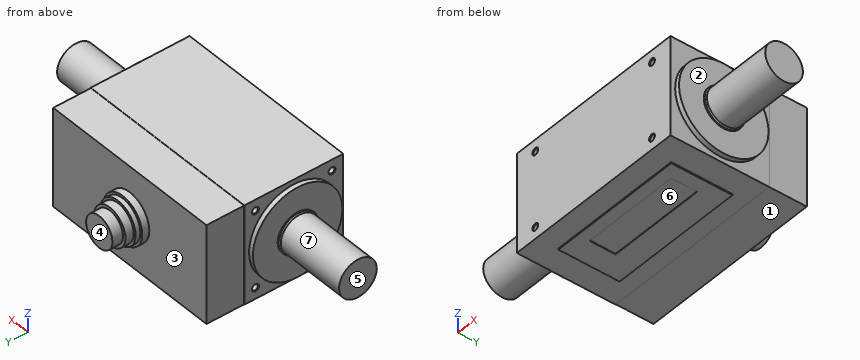
```python
from build123d import *

# Parameters (mm, degrees)
SKETCH1_W                = 79
SKETCH1_H                = 42
BOSS_EXTRUDE1_DEPTH      = 42
SKETCH2_W                = 78.8
SKETCH2_H                = 41.8
BOSS_EXTRUDE2_DEPTH      = 16
SKETCH3_W                = 58
SKETCH3_H                = 26
BOSS_EXTRUDE3_DEPTH      = 0.5
SKETCH4_W                = 42
SKETCH4_H                = 11
CUT_EXTRUDE1_DEPTH       = 0.25
M2_CLEARANCE_HOLE1_D     = 2.459
M2_CLEARANCE_HOLE1_DEPTH = 6.9
M2_CLEARANCE_HOLE1_TIP   = 0.709852156
M2_CLEARANCE_HOLE2_D     = 2.459
M2_CLEARANCE_HOLE2_DEPTH = 7.2
M2_CLEARANCE_HOLE2_TIP   = 0.709852156
CHAMFER1_SIZE            = 0.2705


with BuildPart() as part:
    # Sketch1 → Boss-Extrude1 (new body)
    with BuildSketch(Plane(origin=(0, 21, 0), x_dir=(1, 0, 0), z_dir=(0, 1, 0))):
        Rectangle(SKETCH1_W, SKETCH1_H)
    extrude(amount=-BOSS_EXTRUDE1_DEPTH)

    # Sketch2 → Boss-Extrude2 (add)
    with BuildSketch(Plane(origin=(0, 21, 0), x_dir=(-1, 0, 0), z_dir=(0, 1, 0))):
        Rectangle(SKETCH2_W, SKETCH2_H)
    extrude(amount=BOSS_EXTRUDE2_DEPTH)

    # Sketch3 → Boss-Extrude3 (add)
    with BuildSketch(Plane(origin=(0, 0, -21), x_dir=(-1, 0, 0), z_dir=(0, 0, -1))):
        with Locations((0, 1)):
            Rectangle(SKETCH3_W, SKETCH3_H)
    extrude(amount=BOSS_EXTRUDE3_DEPTH)

    # Sketch4 → Cut-Extrude1 (cut)
    with BuildSketch(Plane(origin=(0, 0, -21.5), x_dir=(-1, 0, 0), z_dir=(0, 0, -1))):
        with Locations((-2, -1.5)):
            Rectangle(SKETCH4_W, SKETCH4_H)
    extrude(amount=-CUT_EXTRUDE1_DEPTH, mode=Mode.SUBTRACT)

    # Sketch5 → Revolve1 (revolve)
    with BuildSketch(Plane(origin=(0, 0, 0), x_dir=(-1, 0, 0), z_dir=(0, 0, -1)), mode=Mode.PRIVATE) as revolve1_sk:
        Polygon((-10, 37), (0, 37), (0, 50), (-6.75, 50), (-6.75, 45.5), (-8, 45.5), (-8, 42), (-9, 42), (-9, 40), (-10, 40), align=None)
    revolve(revolve1_sk.sketch.rotate(Axis((0, 37, 0), (0, 1, 0)), 270), axis=Axis((0, 37, 0), (0, 1, 0)))

    # Sketch6 → Revolve2 (revolve)
    with BuildSketch(Plane.XY, mode=Mode.PRIVATE) as revolve2_sk:
        Polygon((39.5, 19), (39.5, 0), (72.5, 0), (72.5, 8), (42.5, 8), (42, 8.5), (41.5, 8.5), (41.5, 19), align=None)
    revolve(revolve2_sk.sketch.rotate(Axis((39.5, 0, 0), (1, 0, 0)), 270), axis=Axis((39.5, 0, 0), (1, 0, 0)))

    # Sketch7 → Revolve3 (revolve)
    with BuildSketch(Plane.XY, mode=Mode.PRIVATE) as revolve3_sk:
        Polygon((-72.5, 8), (-72.5, 0), (-39.5, 0), (-39.5, 19), (-41.5, 19), (-41.5, 8.5), (-42, 8.5), (-42.5, 8), align=None)
    revolve(revolve3_sk.sketch.rotate(Axis((-72.5, 0, 0), (1, 0, 0)), 270), axis=Axis((-72.5, 0, 0), (1, 0, 0)))

    # M2 Clearance Hole1
    with Locations(Plane.ZY.offset(39.5)):
        with Locations((-16.263455967, 16.263455967), (16.263455967, 16.263455967), (16.263455967, -16.263455967), (-16.263455967, -16.263455967)):
            Hole(M2_CLEARANCE_HOLE1_D / 2, depth=M2_CLEARANCE_HOLE1_DEPTH)
            with Locations((0, 0, -(M2_CLEARANCE_HOLE1_DEPTH + M2_CLEARANCE_HOLE1_TIP / 2))):  # 120° drill point
                Cone(0, M2_CLEARANCE_HOLE1_D / 2, M2_CLEARANCE_HOLE1_TIP, mode=Mode.SUBTRACT)

    # M2 Clearance Hole2
    with Locations(Plane.XZ.offset(21)):
        with Locations((30, 16), (-30, 16), (30, -16), (-30, -16)):
            Hole(M2_CLEARANCE_HOLE2_D / 2, depth=M2_CLEARANCE_HOLE2_DEPTH)
            with Locations((0, 0, -(M2_CLEARANCE_HOLE2_DEPTH + M2_CLEARANCE_HOLE2_TIP / 2))):  # 120° drill point
                Cone(0, M2_CLEARANCE_HOLE2_D / 2, M2_CLEARANCE_HOLE2_TIP, mode=Mode.SUBTRACT)

    # Chamfer1
    chamfer1_edges = [part.edges().sort_by_distance(p)[0] for p in [
        (-28.7705, -21, 16),
        (31.2295, -21, 16),
        (-39.5, -16.263455967, -15.033955967),
        (-39.5, -16.263455967, 17.492955967),
        (-39.5, 16.263455967, 17.492955967),
        (-39.5, 16.263455967, -15.033955967),
        (-28.7705, -21, -16),
        (31.2295, -21, -16),
    ]]
    chamfer(chamfer1_edges, length=CHAMFER1_SIZE)


solid = part.part
```
Geometry check sheet. Reference: the model listing, model coordinates, mm. Face numbers are marked on the shaded views. A direction names the side the tool comes from. Give positions to 0.01 mm unless a question says otherwise; leave off trailing zeros. Order: outer loops, then holes, each group sorted by start corner. A loop starts at its lowest first (then second) coordinate and runs counter-clockwise, first axis right, second up.
1. Section check B-B, the plane y = 29.5. Enter the section's corners in (x, z).
2. Access from +Z, -Z, +X, -X, +Y, -Y to the whole of each face (thin tool, end or side, straight path). Record for the marked faces 1, 2 and 3.
3. Section check A-A, the plane x = 13. Enter the section's corners in (y, z).
4. Section check C-C, the plane x = 35. Enter the section's corners in (y, z).
5. Release check for a two-part mould opening along Y. For the marked faces 4, 5, 6 and 7 record: pulls with the +Y half, pulls with the -Y half, needs draft (parallel to the pull), parting line crosses it, or undercut.
6. Gauge pin test, flat ends, axial feed: pin 1 Ø12 at (x, z) = (-55, -13) entering from +Y; pin 2 Ø2 at (x, z) = (17, -13) entering from +Y; pin 3 Ø1 at (x, y) = (-18, 21) entering from -Z. Record the tip position at first contact, or that the pin passes through.
7. Thickness scan on L1, parallel to Z at x = -30, y = -17.5; L2, parallel to X at y = -18, z = 16; L3, parallel to Z at x = 17.5, y = -14. Record the ranges inside material, lowest first.
Values follow:
1. outline: (-39.4, -20.9) - (39.4, -20.9) - (39.4, 20.9) - (-39.4, 20.9) - close
2. face 1: -Z, +X, -X, +Y
2. face 2: +X
2. face 3: +Y
3. outline: (-21, -21) - (-12, -21) - (-12, -21.5) - (-7, -21.5) - (-7, -21.25) - (4, -21.25) - (4, -21.5) - (14, -21.5) - (14, -21) - (21, -21) - (21, -20.9) - (37, -20.9) - (37, 20.9) - (21, 20.9) - (21, 21) - (-21, 21) - close
4. outline: (-21, -21) - (21, -21) - (21, -20.9) - (37, -20.9) - (37, 20.9) - (21, 20.9) - (21, 21) - (-21, 21) - close
5. face 4: pulls with the +Y half
5. face 5: needs draft
5. face 6: undercut
5. face 7: parting line crosses it
6. pin 1: stops at y = 3.87
6. pin 2: stops at y = 37
6. pin 3: stops at z = -21
7. L1: z = -21 to -17.23, -14.77 to 14.77, 17.23 to 21
7. L2: x = -39.5 to -31.23, -28.77 to 28.77, 31.23 to 39.5
7. L3: z = -21 to 21
